from build123d import *

# Parameters (mm, degrees)
F0_W           = 450
F0_H           = 450
F1_DEPTH       = 15
F3_D           = 17.5
F3_DEPTH       = 57.5
F3_CSINK_D     = 42
F3_CSINK_ANGLE = 90
F3_TIP         = 5.2575304165
F4_SIZE        = 50


with BuildPart() as f1:
    # F0 (on Top) → F1 (new body)
    with BuildSketch(Plane.XY):
        Rectangle(F0_W, F0_H)
    extrude(amount=F1_DEPTH)

    # F3
    with Locations(Plane.XY.offset(15)):
        with Locations((169.7056274848, 169.7056274848), (169.7056274848, -169.7056274848), (-169.7056274848, -169.7056274848), (-169.7056274848, 169.7056274848), (-106.066017178, 106.066017178), (106.066017178, 106.066017178), (106.066017178, -106.066017178), (-106.066017178, -106.066017178)):
            CounterSinkHole(F3_D / 2, F3_CSINK_D / 2, depth=F3_DEPTH, counter_sink_angle=F3_CSINK_ANGLE)
            with Locations((0, 0, -(F3_DEPTH + F3_TIP / 2))):  # 118° drill point
                Cone(0, F3_D / 2, F3_TIP, mode=Mode.SUBTRACT)

    # F4
    f4_edges = [f1.edges().sort_by_distance(p)[0] for p in [
        (225, -225, 7.5),
        (225, 225, 7.5),
        (-225, 225, 7.5),
        (-225, -225, 7.5),
    ]]
    chamfer(f4_edges, length=F4_SIZE)


solid = f1.part
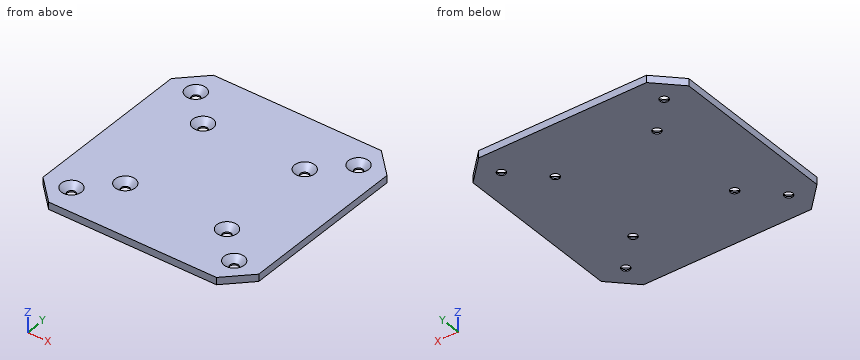
The listing builds one solid part. Answer for the finished solid, in the listing's coordinates (mm). Round coordinates to 2 decimals unless told otherwise and drop trailing zeros. Write each question's results on one line, items separated by ' | '. Start each with the question number.
Item 1: Straight lines are drawn through the part: probe 1 along Y at (x, z) = (-111, 1.75); probe 2 along Y at (x, z) = (163.5, 1.25); probe 3 along X at (y, z) = (182.5, 8.25). For each, find the intervals that lie inside material, in ascending order.
Item 2: Find section A-A on z = 10. Give the number of separate pieces and of enclosed holes in the cut face, and give its area (3 significant figures).
Item 3: Given pin 1 Ø14 at (x, y) = (106.07, 106.07) entering from -Z; pin 2 Ø23 at (x, y) = (-169.71, -169.71) entering from +Z; pin 3 Ø10 at (x, y) = (-41, 64) entering from -Z; pin 4 Ø20 at (x, y) = (-106.07, 106.07) entering from +Z, each flat-ended and moving along its own axis, determine where each tip first touches the part or whether it passes through.
Answer block:
1) probe 1: y = -225 to -113.29, -98.84 to 98.84, 113.29 to 225 | probe 2: y = -225 to -175.87, -163.54 to 163.54, 175.87 to 225 | probe 3: x = -217.5 to -175.98, -163.43 to 163.43, 175.98 to 217.5
2) separate pieces: 1 | enclosed holes: 8 | area: 191,000 mm²
3) pin 1: passes through | pin 2: stops at z = 5.51 | pin 3: stops at z = 0 | pin 4: stops at z = 4.01
